Design review of the part built by this model. Coordinates are the model's own, in mm. Face numbers are marked on the shaded views. A direction names the side the tool comes from. Give positions to 0.01 mm unless a question says otherwise; leave off trailing zeros. Order: outer loops, then holes, each group sorted by start corner. A loop starts at its lowest first (then second) coordinate and runs counter-clockwise, first axis right, second up. Notation, with made-up numbers: (79.25, -12.75) -> (96.25, -12.75) arc R8 cw to (96.25, -6.75) -> close; hole circle Ø1 at (24, 79). An arc over 180 degrees is marked (long way). Return JSON: item names as keys, results as strings.
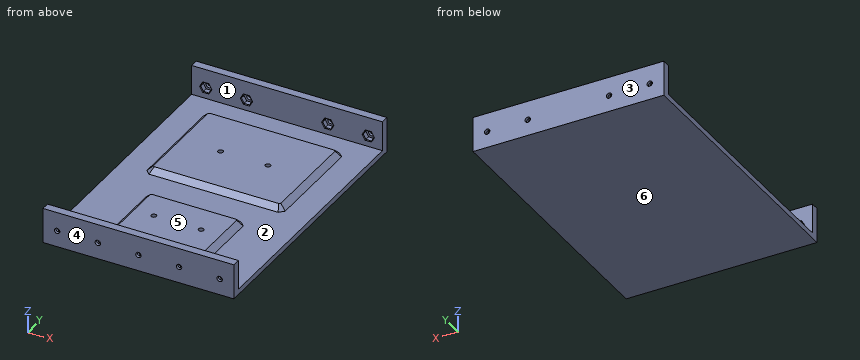
```python
from build123d import *

# Parameters (mm, degrees)
SKETCH1_W               = 140.9
SKETCH1_H               = 204
BOSS_EXTRUDE1_DEPTH     = 4
SKETCH4_W               = 140.9
SKETCH4_H               = 6
BOSS_EXTRUDE3_DEPTH     = 22
CUT_EXTRUDE1_DEPTH      = 217.940550612
CUT_EXTRUDE1_DEPTH_BACK = 217.940550612
SKETCH5_R               = 2
CUT_EXTRUDE4_DEPTH      = 4
SKETCH9_R               = 2
CUT_EXTRUDE5_DEPTH      = 212.308311479
CUT_EXTRUDE6_DEPTH      = 4
CHAMFER1_SIZE           = 0.5
SKETCH11_W              = 64
SKETCH11_H              = 44
SKETCH11_W_2            = 94
SKETCH11_H_2            = 74
BOSS_EXTRUDE4_DEPTH     = 4
CHAMFER2_SIZE           = 1
CHAMFER3_SIZE           = 4
SKETCH12_R              = 1.95
CUT_EXTRUDE7_DEPTH      = 5


with BuildPart() as part:
    # Sketch1 → Boss-Extrude1 (new body)
    with BuildSketch(Plane.XY):
        Rectangle(SKETCH1_W, SKETCH1_H)
    extrude(amount=-BOSS_EXTRUDE1_DEPTH)

    # Sketch4 → Boss-Extrude3 (add)
    with BuildSketch(Plane.XY):
        with Locations((0, 99)):
            Rectangle(SKETCH4_W, SKETCH4_H)
        with Locations((0, -99)):
            Rectangle(SKETCH4_W, SKETCH4_H)
    extrude(amount=BOSS_EXTRUDE3_DEPTH)

    # Sketch5 → Cut-Extrude1 (cut, two sides: drawn at the far end of the back side and taken through both)
    with BuildSketch(Plane(origin=(0, 102, 0), x_dir=(1, 0, 0), z_dir=(0, 1, 0)).offset(-CUT_EXTRUDE1_DEPTH_BACK)):
        with Locations(Location((-30, -8, 0), (0, 0, 270))):
            Circle(SKETCH5_R)
        with Locations(Location((-60, -8, 0), (0, 0, 270))):
            Circle(SKETCH5_R)
        with Locations(Location((60, -8, 0), (0, 0, 90))):
            Circle(SKETCH5_R)
        with Locations(Location((30, -8, 0), (0, 0, 90))):
            Circle(SKETCH5_R)
    extrude(amount=CUT_EXTRUDE1_DEPTH + CUT_EXTRUDE1_DEPTH_BACK, mode=Mode.SUBTRACT)

    # Sketch8 → Cut-Extrude4 (cut)
    with BuildSketch(Plane(origin=(0, -96, 0), x_dir=(1, 0, 0), z_dir=(0, 1, 0))):
        Polygon((-26.016283143, -8), (-28.008141571, -4.55), (-31.991858429, -4.55), (-33.983716857, -8), (-31.991858429, -11.45), (-28.008141571, -11.45), align=None)
        Polygon((-56.016283143, -8), (-58.008141571, -4.55), (-61.991858429, -4.55), (-63.983716857, -8), (-61.991858429, -11.45), (-58.008141571, -11.45), align=None)
        Polygon((33.983716857, -8), (31.991858429, -4.55), (28.008141571, -4.55), (26.016283143, -8), (28.008141571, -11.45), (31.991858429, -11.45), align=None)
        Polygon((63.983716857, -8), (61.991858429, -4.55), (58.008141571, -4.55), (56.016283143, -8), (58.008141571, -11.45), (61.991858429, -11.45), align=None)
    cut_extrude4 = extrude(amount=-CUT_EXTRUDE4_DEPTH, mode=Mode.SUBTRACT)

    # Mirror1: Cut-Extrude4 across plane
    add(cut_extrude4.mirror(Plane.ZX), mode=Mode.SUBTRACT)

    # Sketch9 → Cut-Extrude5 (cut, through all)
    with BuildSketch(Plane(origin=(0, -96, 0), x_dir=(1, 0, 0), z_dir=(0, 1, 0))):
        with Locations(Location((0, -8, 0), (0, 0, 270))):
            Circle(SKETCH9_R)
    extrude(amount=-CUT_EXTRUDE5_DEPTH, mode=Mode.SUBTRACT)

    # Sketch10 → Cut-Extrude6 (cut)
    with BuildSketch(Plane(origin=(0, -96, 0), x_dir=(1, 0, 0), z_dir=(0, 1, 0))):
        Polygon((1.991858429, -4.55), (-1.991858429, -4.55), (-3.983716857, -8), (-1.991858429, -11.45), (1.991858429, -11.45), (3.983716857, -8), align=None)
    extrude(amount=-CUT_EXTRUDE6_DEPTH, mode=Mode.SUBTRACT)

    # Chamfer1
    chamfer1_edges = [part.edges().sort_by_distance(p)[0] for p in [
        (32.987787643, -96, 9.725),
        (32.987787643, -96, 6.275),
        (30, -96, 4.55),
        (27.012212357, -96, 6.275),
        (27.012212357, -96, 9.725),
        (30, -96, 11.45),
        (62.987787643, -96, 9.725),
        (62.987787643, -96, 6.275),
        (60, -96, 4.55),
        (57.012212357, -96, 6.275),
        (57.012212357, -96, 9.725),
        (60, -96, 11.45),
        (-57.012212357, 96, 9.725),
        (-57.012212357, 96, 6.275),
        (-60, 96, 4.55),
        (-62.987787643, 96, 6.275),
        (-62.987787643, 96, 9.725),
        (-60, 96, 11.45),
        (-27.012212357, 96, 9.725),
        (-27.012212357, 96, 6.275),
        (-30, 96, 4.55),
        (-32.987787643, 96, 6.275),
        (-32.987787643, 96, 9.725),
        (-30, 96, 11.45),
        (32.987787643, 96, 9.725),
        (32.987787643, 96, 6.275),
        (30, 96, 4.55),
        (27.012212357, 96, 6.275),
        (27.012212357, 96, 9.725),
        (30, 96, 11.45),
        (62.987787643, 96, 9.725),
        (62.987787643, 96, 6.275),
        (60, 96, 4.55),
        (57.012212357, 96, 6.275),
        (57.012212357, 96, 9.725),
        (60, 96, 11.45),
        (2.987787643, -96, 6.275),
        (0, -96, 4.55),
        (-2.987787643, -96, 6.275),
        (-2.987787643, -96, 9.725),
        (0, -96, 11.45),
        (2.987787643, -96, 9.725),
        (-57.012212357, -96, 9.725),
        (-57.012212357, -96, 6.275),
        (-60, -96, 4.55),
        (-62.987787643, -96, 6.275),
        (-62.987787643, -96, 9.725),
        (-60, -96, 11.45),
        (-27.012212357, -96, 9.725),
        (-27.012212357, -96, 6.275),
        (-30, -96, 4.55),
        (-32.987787643, -96, 6.275),
        (-32.987787643, -96, 9.725),
        (-30, -96, 11.45),
    ]]
    chamfer(chamfer1_edges, length=CHAMFER1_SIZE)

    # Sketch11 → Boss-Extrude4 (add)
    with BuildSketch(Plane.XY):
        with Locations((0, -50)):
            Rectangle(SKETCH11_W, SKETCH11_H)
        with Locations((0, 39)):
            Rectangle(SKETCH11_W_2, SKETCH11_H_2)
    extrude(amount=BOSS_EXTRUDE4_DEPTH)

    # Chamfer2
    chamfer2_edges = [part.edges().sort_by_distance(p)[0] for p in [
        (-32, -28, 2),
        (-32, -72, 2),
        (32, -72, 2),
        (32, -28, 2),
        (-47, 76, 2),
        (-47, 2, 2),
        (47, 2, 2),
        (47, 76, 2),
    ]]
    chamfer(chamfer2_edges, length=CHAMFER2_SIZE)

    # Chamfer3
    chamfer3_edges = [part.edges().sort_by_distance(p)[0] for p in [
        (-46.5, 2.5, 0),
        (0, 2, 0),
        (46.5, 2.5, 0),
        (47, 39, 0),
        (46.5, 75.5, 0),
        (0, 76, 0),
        (-46.5, 75.5, 0),
        (-47, 39, 0),
        (-31.5, -71.5, 0),
        (0, -72, 0),
        (31.5, -71.5, 0),
        (32, -50, 0),
        (31.5, -28.5, 0),
        (0, -28, 0),
        (-31.5, -28.5, 0),
        (-32, -50, 0),
    ]]
    chamfer(chamfer3_edges, length=CHAMFER3_SIZE - 0.0001)  # a hair under: the kernel refuses the full size

    # Sketch12 → Cut-Extrude7 (cut)
    with BuildSketch(Plane.XY.offset(4)):
        with Locations((-17.5, 39)):
            Circle(SKETCH12_R)
        with Locations((17.5, 39)):
            Circle(SKETCH12_R)
        with Locations((-17.5, -50)):
            Circle(SKETCH12_R)
        with Locations((17.5, -50)):
            Circle(SKETCH12_R)
    extrude(amount=-CUT_EXTRUDE7_DEPTH, mode=Mode.SUBTRACT)


solid = part.part
```
Item 1: Add section A-A (z = 17.5). Give the boundary of the cut face in (x, y), plus the area to 3 significant figures.
Result set:
{"outline": "(-70.45, -102) -> (70.45, -102) -> (70.45, -96) -> (-70.45, -96) -> close; (-70.45, 96) -> (70.45, 96) -> (70.45, 102) -> (-70.45, 102) -> close", "area": "1,690 mm^2"}
Item 2: Add section D-D (y = -13). Give the boundary of the cut face in (x, z).
Result set:
{"outline": "(-70.45, -4) -> (70.45, -4) -> (70.45, 0) -> (-70.45, 0) -> close"}
Item 3: Mouldability with a two-part tool opening along Y and no side actions: class the marked faces 4, 5 and 6 as released by +Y, released by -Y, zero draft, split by the parting line, or undercut.
Result set:
{"face 4": "released by -Y", "face 5": "undercut", "face 6": "zero draft"}
Item 4: Wall thickness on L1, parallel to X at y = -101, z = 8; L2, parallel to X at y = 101.4, z = 8; L3, parallel to Y at x = -46.5, z = 6.25: over which ranges is each line inside the solid? List them lowest first. Write a range as [from, to].
Result set:
{"L1": "x = [-70.45, -62], [-58, -32], [-28, -2], [2, 28], [32, 58], [62, 70.45]", "L2": "x = [-70.45, -62], [-58, -32], [-28, 28], [32, 58], [62, 70.45]", "L3": "y = [-102, -96], [96, 102]"}
Item 5: Machinability: for the marked faces 1, 2 and 3, which of the approach directions +Z, -Z, +X, -X, +Y, -Y give a long, thin tool a straight path to every point of the face, cutting with its end or side? Answer none if there is none.
Result set:
{"face 1": "+Z, +X, -X", "face 2": "+Z", "face 3": "+Z, -Z, +X, -X, +Y"}
Item 6: For pin 1 (2 mm diameter, centred on x = 29, y = 38.5, fed in from +Z); pin 2 (3 mm diameter, centred on x = -30, z = 8, fed in from +Y); pin 3 (4 mm diameter, centred on x = -38.5, y = -76, fed in from +Z), all flat-tipped, find the tip position at first contact; note any pin that passes through.
Result set:
{"pin 1": "stops at z = 4", "pin 2": "passes through", "pin 3": "stops at z = 0"}
